Geometry check sheet. Reference: the model listing, model coordinates, mm. A direction names the side the tool comes from. Give positions to 0.01 mm unless a question says otherwise; leave off trailing zeros. Write each loop counter-clockwise with the first axis right and the second up, starting at its lowest first coordinate (ties: lowest second). Pieces come first, ordered by that corner, then holes. Notation, with made-up numbers: (-11, -37.5) -> (-6, -37.5) arc R19 cw to (-6, -31.5) -> close; hole circle Ø6 at (18.25, -15). An arc over 180 degrees is marked (long way). Write item = value, one per line. Start each with the question number.
1. Cross-section at A-A, the plane y = -25. Record the cut outline in (x, z).
2. Thickness scan on line 1 along X through (y, z) = (-14, 0); line 2 along X through (y, z) = (-25, 0); line 3 along Y through (x, z) = (29, 0). Record the ranges inside material, lowest first.
3. Set-up check for faces 1 (the cylindrical face through (97.93, -22.07, -0.65)), 2 (the flat face through (3, 0, 0)): record each of +Z, -Z, +X, -X, +Y, -Y from which the full face is reachable in a straight line by a thin tool's end or side.
4. Cross-section at D-D, the plane z = -9. Record the cut outline in (x, y).
5. Cross-section at C-C, the plane x = 43.5. Record the cut outline in (y, z).
6. Depth check by flat-ended pin: P1, Ø12, axis at x = 155.5, z = -5, coming from the +Y side; P2, Ø1, axis at y = -45, z = 1.5, coming from the -X side; P3, Ø6, axis at x = 91, z = -5.5, coming from the -Y side; P4, Ø4, axis at x = 0, z = 0, coming from the +Y side (3 decimals). Enter the tip coordinate at first touch or a pass-through.
7. Cross-section at B-B, the plane z = 0. Record the cut outline in (x, y).
8. Mould release check, pull along Z, two halves, no side actions. Record for faces 3 (the cylindrical face through (-5.902, -27.115, 3.763)), 4 (the cylindrical face through (-2.44, -27.12, -0.54)), 5 (the flat face through (3, -55, 0)): pulls with the +Z half, pulls with the -Z half, needs draft (parallel to the pull), parting line crosses it, or undercut.
```python
from build123d import *

# Parameters (mm, degrees)
ESQUISSE1_W             = 7
ESQUISSE1_H             = 55
ESQUISSE2_W             = 70
ESQUISSE2_H             = 3
ESQUISSE3_W             = 2
ESQUISSE3_H             = 1.5
ESQUISSE5_R             = 2.5
ENL_V_MAT_EXTRU_1_DEPTH = 96.052617065
ESQUISSE8_R             = 1.5
BOSS_EXTRU_1_DEPTH      = 2.5
BOSS_EXTRU_1_DEPTH_BACK = 3
ESQUISSE11_R            = 1.5
BOSS_EXTRU_2_DEPTH      = 2.5
BOSS_EXTRU_2_DEPTH_BACK = 3
ESQUISSE12_R            = 3
BOSS_EXTRU_3_DEPTH      = 110
BOSS_EXTRU_3_DEPTH_BACK = 71.5


with BuildPart() as part:
    # Esquisse1 → Révolution1 (revolve)
    with BuildSketch(Plane.XY, mode=Mode.PRIVATE) as r_volution1_sk:
        with Locations((3.5, -27.5)):
            Rectangle(ESQUISSE1_W, ESQUISSE1_H)
    revolve(r_volution1_sk.sketch.rotate(Axis((0, 0, 0), (0, -1, 0)), 90), axis=Axis((0, 0, 0), (0, -1, 0)))

    # Esquisse4 → Révolution5 (revolve)
    with BuildSketch(Plane(origin=(0, 0, 0), x_dir=(0, 0, -1), z_dir=(1, 0, 0)), mode=Mode.PRIVATE) as r_volution5_sk:
        Polygon((6.966968242, -50), (7, -48.5), (9, -48.5), (9, -50), align=None)
    revolve(r_volution5_sk.sketch.rotate(Axis((0, -50, 17.973106255), (0, 0, -1)), 90), axis=Axis((0, -50, 17.973106255), (0, 0, -1)))

    # Esquisse5 → Enlèv. mat.-Extru.1 (cut, through all)
    with BuildSketch(Plane(origin=(0, 0, 0), x_dir=(1, 0, 0), z_dir=(0, 1, 0))):
        with Locations(Location((0, 0, 0), (0, 0, 270))):
            Circle(ESQUISSE5_R)
    extrude(amount=-ENL_V_MAT_EXTRU_1_DEPTH, mode=Mode.SUBTRACT)



with BuildPart() as body_2:
    # Esquisse2 → Révolution2 (revolve)
    with BuildSketch(Plane.XY, mode=Mode.PRIVATE) as r_volution2_sk:
        with Locations((42, -23.5)):
            Rectangle(ESQUISSE2_W, ESQUISSE2_H)
    revolve(r_volution2_sk.sketch.rotate(Axis((-18.358665949, -25, 0), (1, 0, 0)), 90), axis=Axis((-18.358665949, -25, 0), (1, 0, 0)))


with BuildPart() as body_3:
    # Esquisse3 → Révolution4 (revolve)
    with BuildSketch(Plane(origin=(0, 0, 0), x_dir=(0, 0, -1), z_dir=(1, 0, 0)), mode=Mode.PRIVATE) as r_volution4_sk:
        with Locations((-8, -49.25)):
            Rectangle(ESQUISSE3_W, ESQUISSE3_H)
    revolve(r_volution4_sk.sketch.rotate(Axis((0, -50, 15.119555316), (0, 0, -1)), 90), axis=Axis((0, -50, 15.119555316), (0, 0, -1)))


with BuildPart() as part_1:
    add(part.part)

    add(body_3.part)  # Boss.-Extru.1 merges body 3
    # Esquisse8 → Boss.-Extru.1 (add, two sides)
    with BuildSketch(Plane.XY.offset(9)) as boss_extru_1_sk:
        with Locations((0, -50)):
            Circle(ESQUISSE8_R)
    extrude(amount=BOSS_EXTRU_1_DEPTH)
    extrude(boss_extru_1_sk.sketch, amount=-BOSS_EXTRU_1_DEPTH_BACK)

    # Esquisse11 → Boss.-Extru.2 (add, two sides)
    with BuildSketch(Plane(origin=(0, 0, -9), x_dir=(-1, 0, 0), z_dir=(0, 0, -1))) as boss_extru_2_sk:
        with Locations(Location((0, -50, 0), (0, 0, 180))):
            Circle(ESQUISSE11_R)
    extrude(amount=BOSS_EXTRU_2_DEPTH)
    extrude(boss_extru_2_sk.sketch, amount=-BOSS_EXTRU_2_DEPTH_BACK)


    add(body_2.part)  # Boss.-Extru.3 merges body 2
    # Esquisse12 → Boss.-Extru.3 (add, two sides)
    with BuildSketch(Plane(origin=(77, 0, 0), x_dir=(0, 0, -1), z_dir=(1, 0, 0))) as boss_extru_3_sk:
        with Locations(Location((0, -25, 0), (0, 0, 180))):
            Circle(ESQUISSE12_R)
    extrude(amount=BOSS_EXTRU_3_DEPTH)
    extrude(boss_extru_3_sk.sketch, amount=-BOSS_EXTRU_3_DEPTH_BACK)


solid = part_1.part
```
Answers:
q1.outline = (6.32, -3) -> (187, -3) -> (187, 3) -> (6.32, 3) arc R7 ccw (long way) to start; hole circle Ø5 at (0, 0)
q2.line_1 = -7 to -2.5, 2.5 to 7
q2.line_2 = -7 to -2.5, 2.5 to 187
q2.line_3 = -28 to -22
q3.face_1 = +X
q3.face_2 = +Z, -Z, +X, -X, +Y
q4.outline = circle Ø3 at (0, -50)
q5.outline = circle Ø6 at (-25, 0)
q6.P1 = -22
q6.P2 = -6.93
q6.P3 = -26.66
q6.P4 = through
q7.outline = (-7, -55) -> (-2.5, -55) -> (-2.5, 0) -> (-7, 0) -> close; (2.5, -55) -> (7, -55) -> (7, -28) -> (187, -28) -> (187, -22) -> (7, -22) -> (7, 0) -> (2.5, 0) -> close
q8.face_3 = parting line crosses it
q8.face_4 = undercut
q8.face_5 = needs draft
